Here's how the part is built. I have some questions about the finished solid (model axes, mm). Face numbers are marked on the shaded views. A direction names the side the tool comes from. Give positions to 0.01 mm unless a question says otherwise; leave off trailing zeros. Write each loop counter-clockwise with the first axis right and the second up, starting at its lowest first coordinate (ties: lowest second). Pieces come first, ordered by that corner, then holes. Notation, with made-up numbers: M 85.5,4 L 136.5,4 A18 ccw 136.5,26 Z; hole C 73,40 d9. An arc over 180 degrees is marked long. Answer as CSV lines item,"result". Start each with the question number.
Q1. If I drill on line 1 along Y through (x, z) = (-2.5, -2); line 2 along Y through (x, z) = (-2.65, 0); line 3 along X through (y, z) = (5.25, 4.25), over which ranges is the centre line in solid material (lowest first)?
Q2. Suppose I cut it at C-C (x = -5). Write out the boundary of the cut face in (y, z), then the cut area to 3 significant figures.
Q3. Suppose I cut it at B-B (x = -2). Write out the boundary of the cut face in (y, z), then the cut area to 3 significant figures.
Q4. For pin 1 (5 mm diameter, centred on y = 4.5, z = -6.5, fed in from -X); pin 2 (2 mm diameter, centred on x = -4.5, y = 5, fed in from -Z); pin 3 (2 mm diameter, centred on x = -4.5, z = 10.5, fed in from +Y), each with a flat end and sliding along its axis, tell me the tip position at first contact or that it passes through.
Q5. Suppose I cut it at A-A (y = 0). Write out the boundary of the cut face in (x, z).
Q6. On a 3-axis mill with a long thin cutter (end or side, diameter ignored), from which of +Z, -Z, +X, -X, +Y, -Y can I reach the whole of each face in a straight line? I mean the marked faces 1, 2 and 3. Say none if no direction works.
Q7. Thinking about a two-plate mould opening in Z: for the marked faces 4, 5 and 6, which applies, +Z half, -Z half, draft (parallel to the pull), parting line (faces both ways), or undercut?
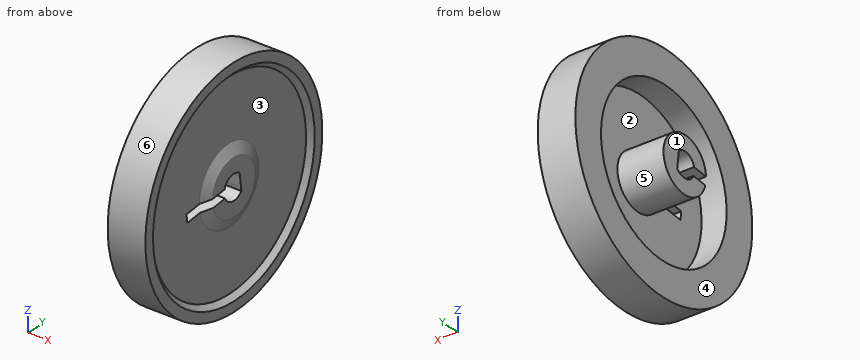
```python
from build123d import *

# Parameters (mm, degrees)
CORTAR_EXTRUIR1_DEPTH = 10


with BuildPart() as part:
    # Croquis1 → Revolución2 (revolve)
    with BuildSketch(Plane.XY, mode=Mode.PRIVATE) as revoluci_n2_sk:
        Polygon((0, 12.334092632), (0, 13.5), (-4.5, 13.5), (-4.5, 9.583549686), (-1.5, 9.583549686), (-1.5, 3.25), (-7, 3.25), (-7, 0), (0, 0), (0, 3.25), (-0.574918787, 4.530302725), (-0.574918787, 11.759173845), align=None)
    revolve(revoluci_n2_sk.sketch.rotate(Axis((-7, 0, 0), (1, 0, 0)), 90), axis=Axis((-7, 0, 0), (1, 0, 0)))

    # Croquis2 → Cortar-Extruir1 (cut)
    with BuildSketch(Plane(origin=(0, 0, 0), x_dir=(0, 0, -1), z_dir=(1, 0, 0))):
        with BuildLine():
            Line((0.916823697, 1.149058009), (0.524737182, 1.101385895))
            Line((0.524737182, 1.101385895), (-0.77337267, 0.943554298))
            Line((-0.77337267, 0.943554298), (-1.165459185, 0.895882184))
            ThreePointArc((-1.165459185, 0.895882184), (-1.392146699, -0.472046151), (-0.380201076, -1.419981388))
            Line((-0.380201076, -1.419981388), (0.236111814, -6.488940003))
            Line((0.236111814, -6.488940003), (1.228801228, -6.368243164))
            Line((1.228801228, -6.368243164), (0.616752973, -1.334359685))
            ThreePointArc((0.616752973, -1.334359685), (1.459385217, -0.176337142), (0.916823697, 1.149058009))
        make_face()
    extrude(amount=-CORTAR_EXTRUIR1_DEPTH, mode=Mode.SUBTRACT)


solid = part.part
```
Resolved:
1,line 1,"-13.35 to -9.37, -2.56 to 2.56, 9.37 to 13.35"
1,line 2,"-13.5 to -9.58, 1.04 to 3.25, 9.58 to 13.5"
1,line 3,"-1.5 to -0.57"
2,outline,"M -3.25,0.16 L -1.42,0.38 A1.47 cw 0.9,1.17 L 1.15,-0.92 A1.47 cw -1.33,-0.62 L -3.14,-0.84 A3.25 ccw long Z"
2,area,"25.2 mm^2"
3,outline,"C 0,0 d27; M -3.25,0.16 L -1.42,0.38 A1.47 cw 0.9,1.17 L 1.15,-0.92 A1.47 cw -1.33,-0.62 L -3.14,-0.84 A3.25 ccw long Z; hole C 0,0 d19.17"
3,area,"309 mm^2"
4,pin 1,"x = -4.5"
4,pin 2,"z = -12.89"
4,pin 3,"y = 9.59"
5,outline,"M -7,-3.25 L -1.5,-3.25 L -1.5,-9.58 L -4.5,-9.58 L -4.5,-13.5 L 0,-13.5 L 0,-12.33 L -0.57,-11.76 L -0.57,-4.53 L 0,-3.25 L 0,-1.47 L -7,-1.47 Z; M -7,1.47 L 0,1.47 L 0,3.25 L -0.57,4.53 L -0.57,11.76 L 0,12.33 L 0,13.5 L -4.5,13.5 L -4.5,9.58 L -1.5,9.58 L -1.5,3.25 L -7,3.25 Z"
6,face 1,"+Z, -Z, -X, +Y, -Y"
6,face 2,"-X"
6,face 3,"+X"
7,face 4,"draft"
7,face 5,"undercut"
7,face 6,"parting line"
